The model under review builds one solid part; all positions refer to its coordinate system, in mm. Coordinates: 2 decimals unless noted, no trailing zeros. Loops run counter-clockwise (first coordinate to the right, second up) from the corner with the lowest first, then second, coordinate; pieces in that order, holes last. Notation, with made-up numbers: M -5,45 L 12,45 A25 cw 12,68 Z; hole C 68,-6 d10. An arc over 180 degrees is marked long. Return JSON: item names as keys, results as strings.
```python
from build123d import *

# Parameters (mm, degrees)
MODEL_R         = 1.5
EXTRUDE_1_DEPTH = 3


with BuildPart() as part:
    # Model → 凸台-拉伸1 (new body)
    with BuildSketch(Plane.XY):
        with BuildLine():
            Line((2493.366322478, 1849.391249913), (2493.366322478, 1609.391249913))
            Line((2493.366322478, 1609.391249913), (2453.366322478, 1609.391249913))
            ThreePointArc((2453.366322478, 1609.391249913), (2449.24094139, 1662.258404711), (2447.449369938, 1715.255999913))
            ThreePointArc((2447.449369938, 1715.255999913), (2448.315416133, 1717.400070674), (2450.449162837, 1718.291249913))
            Line((2450.449162837, 1718.291249913), (2455.366322478, 1718.291249913))
            ThreePointArc((2455.366322478, 1718.291249913), (2457.487642822, 1719.16992957), (2458.366322478, 1721.291249913))
            Line((2458.366322478, 1721.291249913), (2458.366322478, 1737.491249913))
            ThreePointArc((2458.366322478, 1737.491249913), (2457.487642822, 1739.612570257), (2455.366322478, 1740.491249913))
            Line((2455.366322478, 1740.491249913), (2450.449162837, 1740.491249913))
            ThreePointArc((2450.449162837, 1740.491249913), (2448.315416133, 1741.382429153), (2447.449369938, 1743.526499913))
            ThreePointArc((2447.449369938, 1743.526499913), (2449.24094139, 1796.524095116), (2453.366322478, 1849.391249913))
            Line((2453.366322478, 1849.391249913), (2493.366322478, 1849.391249913))
        make_face()
        with Locations((2479.366322478, 1619.891249913)):
            Circle(MODEL_R, mode=Mode.SUBTRACT)
        with Locations((2467.366322478, 1619.891249913)):
            Circle(MODEL_R, mode=Mode.SUBTRACT)
        with Locations((2467.366322478, 1838.891249913)):
            Circle(MODEL_R, mode=Mode.SUBTRACT)
        with Locations((2479.366322478, 1838.891249913)):
            Circle(MODEL_R, mode=Mode.SUBTRACT)
        with Locations((2465.366322478, 1752.491249913)):
            Circle(MODEL_R, mode=Mode.SUBTRACT)
        with Locations((2465.366322478, 1706.291249913)):
            Circle(MODEL_R, mode=Mode.SUBTRACT)
        with Locations((2451.366322478, 1706.291249913)):
            Circle(MODEL_R, mode=Mode.SUBTRACT)
        with Locations((2451.366322478, 1752.491249913)):
            Circle(MODEL_R, mode=Mode.SUBTRACT)
    extrude(amount=EXTRUDE_1_DEPTH)


solid = part.part
```
1. Add section C-C on y = 1659. Give the boundary of the cut face in (x, z), plus the area to 3 significant figures.
Check values:
{"outline": "M 2449.43,0 L 2493.37,0 L 2493.37,3 L 2449.43,3 Z", "area": "132 mm²"}
2. Add section A-A on z = 1.05. State how many separate pieces and enclosed holes the cut face has, plus the area to 3 significant figures.
Check values:
{"separate pieces": "1", "enclosed holes": "8", "area": "10,300 mm²"}
3. To check wall thickness, follow line 1 (Y direction, x = 2465.5, z = 2.75); line 2 (Y direction, x = 2467, z = 2.8); line 3 (Y direction, x = 2454.5, z = 0.9). State the ranges of each line that lie inside material, in increasing order.
Check values:
{"line 1": "1609.39 to 1704.8, 1707.79 to 1751, 1753.99 to 1849.39", "line 2": "1609.39 to 1618.44, 1621.35 to 1837.44, 1840.35 to 1849.39", "line 3": "1609.39 to 1718.29, 1740.49 to 1849.39"}
4. Add section B-B on y = 1731.5. Give the boundary of the cut face in (x, z), plus the area to 3 significant figures.
Check values:
{"outline": "M 2458.37,0 L 2493.37,0 L 2493.37,3 L 2458.37,3 Z", "area": "105 mm²"}
